Geometry check sheet. Reference: drawing and pictorial views, mm from the part's lowest x, y, z. A direction names the side the tool comes from. Round coordinates to 2 decimals unless told otherwise and drop trailing zeros. Write each loop counter-clockwise with the first axis right and the second up, starting at its lowest first coordinate (ties: lowest second). Pieces come first, ordered by that corner, then holes. Notation, with made-up numbers: (34.25, 80.25) - (47.25, 80.25) arc R9 cw to (47.25, 91.25) - close; hole circle Ø5 at (73, 89). An arc over 180 degrees is marked (long way). Use one line per item in the form item = value. Start each with the question number.
1) Set-up check for the marked faces 1, 2 and 3: record each of +Z, -Z, +X, -X, +Y, -Y from which the full face is reachable in a straight line by a thin tool's end or side.
2) Scan lines: probe 1 along Y at (x, z) = (5, 15.25); probe 2 along Y at (x, z) = (6.5, 13); probe 3 along Y at (x, z) = (2.5, 14.25). Record each from-to range of solid material in increasing order.
3) Section check B-B (z = 10). Record the boundary of the cut face in (x, y), then the cut area to 3 significant figures.
4) Section check A-A (x = 6). Record the boundary of the cut face in (y, z).
5) Section check C-C (y = 78). Record the boundary of the cut face in (x, z), then the cut area to 3 significant figures.
6) Gauge pin test, flat ends, axial feed: P1, Ø5, axis at x = 9.5, z = 17.5, coming from the -Y side; P2, Ø2, axis at x = 5.5, y = 117, coming from the +Z side; P3, Ø1.5, axis at x = 3, y = 129.5, coming from the -Z side; P4, Ø1, axis at y = 25, z = 16, coming from the +X side. Record the tip position at first contact, or that the pin passes through.
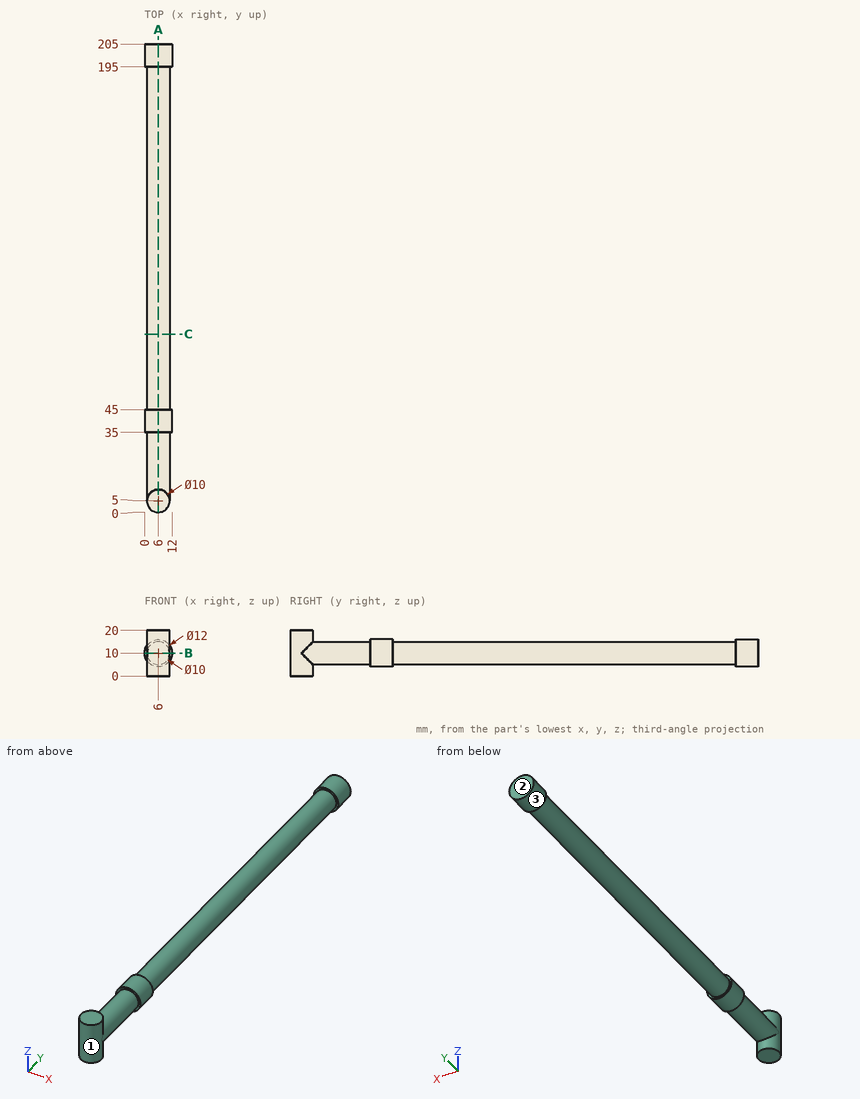
Results are:
q1.face_1 = none
q1.face_2 = +Z, -Z, +X, -X, +Y
q1.face_3 = +Y
q2.probe_1 = 0.1 to 9.9, 35 to 45, 195 to 205
q2.probe_2 = 0.03 to 205
q2.probe_3 = 1.43 to 8.57, 35 to 45, 195 to 205
q3.outline = (0, 35) - (1, 35) - (1, 5) arc R5 ccw to (11, 5) - (11, 35) - (12, 35) - (12, 45) - (11, 45) - (11, 195) - (12, 195) - (12, 205) - (0, 205) - (0, 195) - (1, 195) - (1, 45) - (0, 45) - close
q3.area = 2,080 mm²
q4.outline = (0, 0) - (10, 0) - (10, 5) - (35, 5) - (35, 4) - (45, 4) - (45, 5) - (195, 5) - (195, 4) - (205, 4) - (205, 16) - (195, 16) - (195, 15) - (45, 15) - (45, 16) - (35, 16) - (35, 15) - (10, 15) - (10, 20) - (0, 20) - close
q5.outline = circle Ø10 at (6, 10)
q5.area = 78.5 mm²
q6.P1 = 0.1
q6.P2 = 15
q6.P3 = 5.53
q6.P4 = through
